from build123d import *

# Parameters (mm, degrees)
SKETCH_1_R      = 3.25
SKETCH_1_R_2    = 1.75
EXTRUDE_1_DEPTH = 8


with BuildPart() as part:
    # 草圖1 → 填料-伸長1 (new body)
    with BuildSketch(Plane.XY):
        with BuildLine():
            Line((-5.423089748, 35), (-32.24596582, -35))
            add(Edge.make_bspline(
                [(-32.24596582, -35), (-37, -46), (-25, -45.023391813)],
                knots=[0, 0, 0, 1, 1, 1], degree=2))
            Line((-25, -45.023391813), (25, -45.023391813))
            add(Edge.make_bspline(
                [(32.24596582, -35), (37, -46), (25, -45.023391813)],
                knots=[0, 0, 0, 1, 1, 1], degree=2))
            Line((32.24596582, -35), (5.423089748, 35))
            add(Edge.make_bspline(
                [(-5.423089748, 35), (0, 43.412192281), (5.423089748, 35)],
                knots=[0, 0, 0, 1, 1, 1], degree=2))
        make_face()
        with Locations((0, 30)):
            Circle(SKETCH_1_R, mode=Mode.SUBTRACT)
        with Locations((-28, -40)):
            Circle(SKETCH_1_R, mode=Mode.SUBTRACT)
        with Locations((28, -40)):
            Circle(SKETCH_1_R, mode=Mode.SUBTRACT)
        with Locations((-4.971323351, 25)):
            Circle(SKETCH_1_R_2, mode=Mode.SUBTRACT)
        with Locations((-9.265095937, 13.794487206)):
            Circle(SKETCH_1_R_2, mode=Mode.SUBTRACT)
        with Locations((-13.558868522, 2.588974411)):
            Circle(SKETCH_1_R_2, mode=Mode.SUBTRACT)
        with Locations((-17.852641108, -8.616538383)):
            Circle(SKETCH_1_R_2, mode=Mode.SUBTRACT)
        with Locations((-22.146413694, -19.822051177)):
            Circle(SKETCH_1_R_2, mode=Mode.SUBTRACT)
        with Locations((-26.44018628, -31.027563971)):
            Circle(SKETCH_1_R_2, mode=Mode.SUBTRACT)
        with Locations((-16, -40.523391813)):
            Circle(SKETCH_1_R_2, mode=Mode.SUBTRACT)
        with Locations((-8, -40.523391813)):
            Circle(SKETCH_1_R_2, mode=Mode.SUBTRACT)
        with Locations((0, -40.523391813)):
            Circle(SKETCH_1_R_2, mode=Mode.SUBTRACT)
        with Locations(Location((8, -40.523391813, 0), (0, 0, 180))):
            Circle(SKETCH_1_R_2, mode=Mode.SUBTRACT)
        with Locations(Location((16, -40.523391813, 0), (0, 0, 180))):
            Circle(SKETCH_1_R_2, mode=Mode.SUBTRACT)
        with Locations(Location((26.44018628, -31.027563971, 0), (0, 0, 180))):
            Circle(SKETCH_1_R_2, mode=Mode.SUBTRACT)
        with Locations(Location((22.146413694, -19.822051177, 0), (0, 0, 180))):
            Circle(SKETCH_1_R_2, mode=Mode.SUBTRACT)
        with Locations(Location((17.852641108, -8.616538383, 0), (0, 0, 180))):
            Circle(SKETCH_1_R_2, mode=Mode.SUBTRACT)
        with Locations(Location((13.558868522, 2.588974411, 0), (0, 0, 180))):
            Circle(SKETCH_1_R_2, mode=Mode.SUBTRACT)
        with Locations(Location((9.265095937, 13.794487206, 0), (0, 0, 180))):
            Circle(SKETCH_1_R_2, mode=Mode.SUBTRACT)
        with Locations(Location((4.971323351, 25, 0), (0, 0, 180))):
            Circle(SKETCH_1_R_2, mode=Mode.SUBTRACT)
        Polygon((0, 24), (-23, -36.023391813), (23, -36.023391813), align=None, mode=Mode.SUBTRACT)
    extrude(amount=EXTRUDE_1_DEPTH)


solid = part.part
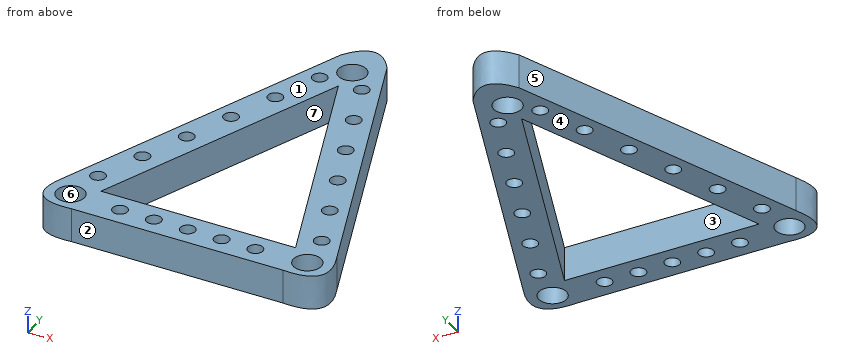
Input: part model. Units: mm. Frame: model coordinates. Face numbers are marked on the shaded views. A direction names the side the tool comes from. Round coordinates to 2 decimals unless told otherwise and drop trailing zeros. Order: outer loops, then holes, each group sorted by start corner. A loop starts at its lowest first (then second) coordinate and runs counter-clockwise, first axis right, second up. Notation, with made-up numbers: (56.5, 25) - (109.5, 25) arc R26 ccw to (109.5, 50) - close; hole circle Ø6 at (48, 30). An arc over 180 degrees is marked (long way). Answer as a JSON object with one key per item and string values. Group by question number.
(1) Cut plane B-B (y = 30). Return loops of the section in (x, z), then the cut area to 3 significant figures.
(2) Reachability of the marked faces 1, 2 and 3 from +Z, -Z, +X, -X, +Y, -Y: full face, straight path, thin tool, end or side. Return the list, or none.
(3) Pin query (flat end, axial travel): P1, Ø3, axis at x = 22.15, y = -19.82, coming from the +Z side; P2, Ø1.5, axis at y = -18.5, z = 2, coming from the +X side; P3, Ø2, axis at y = -1, z = 4.5, coming from the -X side; P4, Ø3, axis at y = -5.5, z = 2, coming from the -X side. Return the tip coordinate at first contact, or that it passes through.
(4) Material intervals for probe 1 along X at (y, z) = (3, 2.5); probe 2 along X at (y, z) = (14, 3); probe 3 along X at (y, z) = (21, 3.5), sorted ascending. Write a range as from..to.
(5) Cut plane A-A (x = -13). Return loops of the section in (y, z).
(6) Draft query along Y for the marked faces 4, 5, 6 and 7. Return one class per face: released by +Y, released by -Y, zero draft, split by the parting line, or undercut.
(7) Cut plane C-C (z = 2.25). Count the separate pieces of the cut face and the enclosed holes in it, then the cut area to 3 significant figures.
Here are the results:
{
 "1": {"outline": "(-7.34, 0) - (-3.25, 0) - (-3.25, 8) - (-7.34, 8) - close; (3.25, 0) - (7.34, 0) - (7.34, 8) - (3.25, 8) - close", "area": "65.4 mm^2"},
 "2": {"face 1": "+Z, +X, -X, +Y, -Y", "face 2": "+Z, -Z, -Y", "face 3": "+Z, -Z"},
 "3": {"P1": "passes through", "P2": "stops at x = 26.21", "P3": "stops at x = -19.6", "P4": "stops at x = -21.52"},
 "4": {"probe 1": "x = -17.68..-15.26, -11.86..-8.05, 8.05..11.86, 15.26..17.68", "probe 2": "x = -13.47..-11, -7.53..-3.83, 3.83..7.53, 11..13.47", "probe 3": "x = -10.79..-1.15, 1.15..10.79"},
 "5": {"outline": "(-45.02, 0) - (-36.02, 0) - (-36.02, 8) - (-45.02, 8) - close; (-9.93, 0) - (0.93, 0) - (0.93, 8) - (-9.93, 8) - close; (4.25, 0) - (15.23, 0) - (15.23, 8) - (4.25, 8) - close"},
 "6": {"face 4": "zero draft", "face 5": "released by +Y", "face 6": "undercut", "face 7": "undercut"},
 "7": {"separate pieces": "1", "enclosed holes": "21", "area": "1,680 mm^2"}
}
